Geometry check sheet. Reference: the model listing, model coordinates, mm. Round coordinates to 2 decimals unless told otherwise and drop trailing zeros. Order: outer loops, then holes, each group sorted by start corner. A loop starts at its lowest first (then second) coordinate and runs counter-clockwise, first axis right, second up. Notation, with made-up numbers: (-22.5, -30) - (33.5, -30) arc R34 cw to (33.5, 1) - close; hole circle Ø2 at (-9, 78.5). An arc over 180 degrees is marked (long way). Write each question's results on one line, items separated by ' | '.
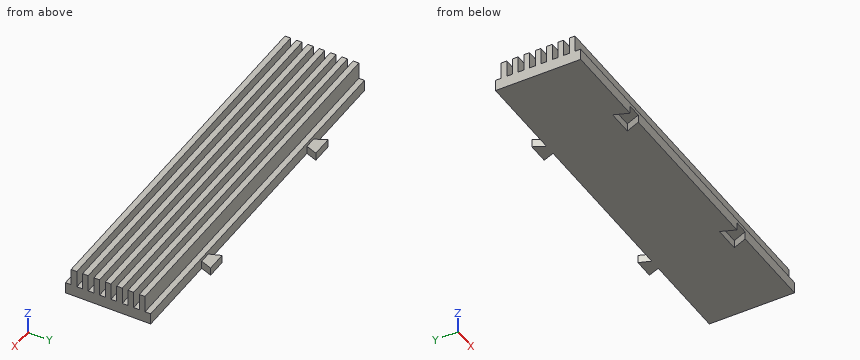
```python
from build123d import *

# Parameters (mm, degrees)
F0_W     = 130
F0_H     = 30
F1_DEPTH = 10
F2_W     = 130
F2_H     = 2
F3_DEPTH = 6
F4_W     = 5
F4_H     = 5
F5_DEPTH = 2.8
F4_W_2   = 4
F4_H_2   = 4
F6_DEPTH = 2.8


with BuildPart() as f1:
    # F0 (on Top) → F1 (new body)
    with BuildSketch(Plane.XY):
        Rectangle(F0_W, F0_H)
    extrude(amount=F1_DEPTH)

    # F2 (on face) → F3 (cut)
    with BuildSketch(Plane.XY.offset(10)):
        with Locations((0, -14)):
            Rectangle(F2_W, F2_H)
        with Locations((0, -10)):
            Rectangle(F2_W, F2_H)
        with Locations((0, -6)):
            Rectangle(F2_W, F2_H)
        with Locations((0, -2)):
            Rectangle(F2_W, F2_H)
        with Locations((0, 2)):
            Rectangle(F2_W, F2_H)
        with Locations((0, 6)):
            Rectangle(F2_W, F2_H)
        with Locations((0, 10)):
            Rectangle(F2_W, F2_H)
        with Locations((0, 14)):
            Rectangle(F2_W, F2_H)
    extrude(amount=-F3_DEPTH, mode=Mode.SUBTRACT)

    # F4 (on face) → F5 (cut)
    with BuildSketch(Plane(origin=(0, 0, 0), x_dir=(1, 0, 0), z_dir=(0, 0, -1))):
        with Locations((-32.5, 12.5)):
            Rectangle(F4_W, F4_H)
        Polygon((-28, 10), (-30, 15), (-30, 10), align=None)
        Polygon((-35, 10), (-35, 15), (-37, 10), align=None)
        with Locations((32.5, 12.5)):
            Rectangle(F4_W, F4_H)
        Polygon((30, 10), (30, 15), (28, 10), align=None)
        Polygon((37, 10), (35, 15), (35, 10), align=None)
    extrude(amount=-F5_DEPTH, mode=Mode.SUBTRACT)

    # F4 (on face) → F6 (join)
    with BuildSketch(Plane(origin=(0, 0, 0), x_dir=(1, 0, 0), z_dir=(0, 0, -1))):
        with Locations((32, -17)):
            Rectangle(F4_W_2, F4_H_2)
        Polygon((35.5, -19), (34, -15), (34, -19), align=None)
        Polygon((30, -19), (30, -15), (28.5, -19), align=None)
        with Locations((-32, -17)):
            Rectangle(F4_W_2, F4_H_2)
        Polygon((-28.5, -19), (-30, -15), (-30, -19), align=None)
        Polygon((-34, -19), (-34, -15), (-35.9975211322, -19), align=None)
    extrude(amount=-F6_DEPTH)


solid = f1.part
```
(1) Material ranges on line 1 (Z direction, x = -36.5, y = -6.5); line 2 (Y direction, x = 41, z = 0.5), recorded low to high.
Answers follow:
line 1: 0 to 4 | line 2: -15 to 15
(2) Depth check by flat-ended pin: pin 1 Ø3 at (x, z) = (-29.5, 7.5) entering from -Y; pin 2 Ø6 at (x, z) = (-6.5, 3.5) entering from +Y; pin 3 Ø3 at (x, z) = (19.5, 6.5) entering from +Y. Enter the tip coordinate at first touch or a pass-through.
Answers follow:
pin 1: y = -13 | pin 2: y = 15 | pin 3: y = 13
(3) Section check B-B (z = 1.5). Record the cut outline in (x, y), then the cut area to 4 significant figures.
Answers follow:
outline: (-65, -15) - (-35, -15) - (-37, -10) - (-28, -10) - (-30, -15) - (30, -15) - (28, -10) - (37, -10) - (35, -15) - (65, -15) - (65, 15) - (34, 15) - (35.5, 19) - (28.5, 19) - (30, 15) - (-30, 15) - (-28.5, 19) - (-36, 19) - (-34, 15) - (-65, 15) - close | area: 3,875 mm²
(4) Section check A-A (z = 7). Record the cut outline in (x, y), then the cut area to 3 significant figures.
Answers follow:
outline: (-65, -13) - (65, -13) - (65, -11) - (-65, -11) - close; (-65, -9) - (65, -9) - (65, -7) - (-65, -7) - close; (-65, -5) - (65, -5) - (65, -3) - (-65, -3) - close; (-65, -1) - (65, -1) - (65, 1) - (-65, 1) - close; (-65, 3) - (65, 3) - (65, 5) - (-65, 5) - close; (-65, 7) - (65, 7) - (65, 9) - (-65, 9) - close; (-65, 11) - (65, 11) - (65, 13) - (-65, 13) - close | area: 1,820 mm²
